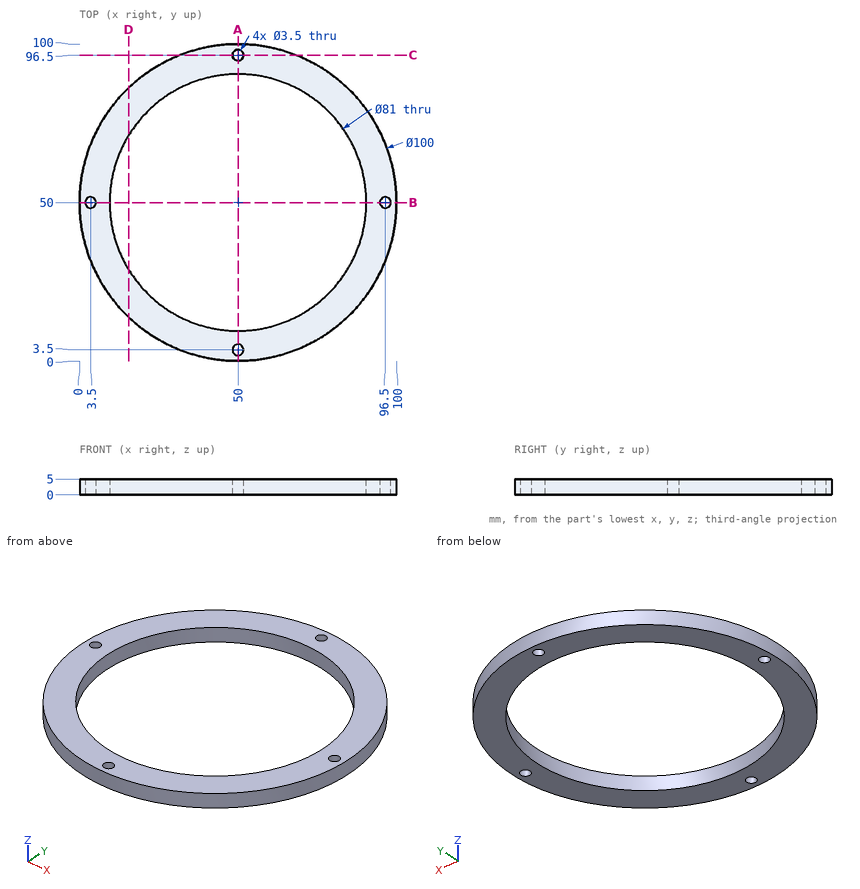
Geometry: see drawing. Coordinates: mm, zero at the bounding-box minimum. Give positions to 0.01 mm unless a question says otherwise; leave off trailing zeros. Order: outer loops, then holes, each group sorted by start corner. A loop starts at its lowest first (then second) coordinate and runs counter-clockwise, first axis right, second up. Notation, with made-up numbers: (51.5, 9.5) - (81.5, 9.5) arc R27 cw to (81.5, 42.5) - close; hole circle Ø3 at (-8.5, 33). An arc over 180 degrees is marked (long way). One line per item, written item: value.
1. Pin query (flat end, axial travel): pin 1 Ø2 at (x, z) = (61.5, 1.5) entering from -Y; pin 2 Ø1.5 at (x, z) = (16, 3.5) entering from -Y; pin 3 Ø5.5 at (x, y) = (3.5, 50) entering from -Z; pin 4 Ø3 at (y, z) = (19.5, 2) entering from -X. Return the tip coordinate at first contact, or that it passes through.
Determined:
pin 1: y = 1.11
pin 2: y = 12.66
pin 3: z = 0
pin 4: x = 9.27
2. Cut plane D-D, the plane x = 15.5. Output: boundary loops of the cut face in (y, z), and give its area (3 significant figures).
Determined:
outline: (13.81, 0) - (28.79, 0) - (28.79, 5) - (13.81, 5) - close; (71.21, 0) - (86.19, 0) - (86.19, 5) - (71.21, 5) - close
area: 150 mm2
3. Cut plane A-A, the plane x = 50. Output: boundary loops of the cut face in (y, z), and give its area (3 significant figures).
Determined:
outline: (0, 0) - (1.75, 0) - (1.75, 5) - (0, 5) - close; (5.25, 0) - (9.5, 0) - (9.5, 5) - (5.25, 5) - close; (90.5, 0) - (94.75, 0) - (94.75, 5) - (90.5, 5) - close; (98.25, 0) - (100, 0) - (100, 5) - (98.25, 5) - close
area: 60.0 mm2
4. Cut plane C-C, the plane y = 96.5. Output: boundary loops of the cut face in (x, z), and give its area (3 significant figures).
Determined:
outline: (31.62, 0) - (48.25, 0) - (48.25, 5) - (31.62, 5) - close; (51.75, 0) - (68.38, 0) - (68.38, 5) - (51.75, 5) - close
area: 166 mm2
5. Line query: probe 1 along Y at (x, z) = (50, 1.45); probe 2 along X at (y, z) = (38, 1.3); probe 3 along X at (y, z) = (57, 2.8). Output: solid intervals per line, ascending.
Determined:
probe 1: 0 to 1.75, 5.25 to 9.5, 90.5 to 94.75, 98.25 to 100
probe 2: 1.46 to 11.32, 88.68 to 98.54
probe 3: 0.49 to 10.11, 89.89 to 99.51
